CAD build for the part. Positions are in the model's coordinates, mm. Coordinates: 2 decimals unless noted, no trailing zeros. Loops run counter-clockwise (first coordinate to the right, second up) from the corner with the lowest first, then second, coordinate; pieces in that order, holes last. Notation, with made-up numbers: (44, 4) -> (86, 4) arc R7 cw to (86, 13) -> close; hole circle Ø6 at (46, 85.25). An arc over 180 degrees is marked (long way). Write item = value, one per line. Start each with the question number.
(1) Drill centre lines: line 1 (X direction, y = 2.3, z = 0); line 2 (Z direction, x = -1, y = 2.5); line 3 (Z direction, x = -0.25, y = 3.65). Where is each one in solid material? Low to high. Write a range as from..to.
(2) Band-saw the part on B-B (z = 0). Write the cut outline in (x, y).
(3) Band-saw the part on C-C (y = 0.55). Write the cut outline in (x, z).
(4) Band-saw the part on D-D (y = 1.75). Write the cut outline in (x, z), and give its area (3 significant figures).
(5) Flat gauge pins, fed straight in: P1, Ø1.5, axis at x = 1.5, y = 2.5, coming from the +Z side; P2, Ø1, axis at x = -2, y = 2.5, coming from the -Z side. Where does each tip first touch, or does it go through?
(6) Band-saw the part on A-A (x = 0). Write the cut outline in (y, z).
(7) Pull direction X, two halves, no side cores. Call faces 1 (the face through (0.45, 2.92, -1.43)), 2 (the face through (-1.4, 2.98, -3.37)): +X half, -X half, draft (parallel to the pull), parting line (faces both ways), or undercut.
```python
from build123d import *


with BuildPart() as part:
    # Sketch1 → Revolve1 (revolve)
    with BuildSketch(Plane.XY, mode=Mode.PRIVATE) as revolve1_sk:
        with BuildLine():
            Line((1.5, 4.9), (1.5, 1))
            ThreePointArc((1.5, 1), (1.792893219, 0.292893219), (2.5, 0))
            Line((2.5, 0), (2.65, 0))
            ThreePointArc((2.65, 0), (3.357106781, 0.292893219), (3.65, 1))
            Line((3.65, 1), (3.65, 4.9))
            ThreePointArc((3.65, 4.9), (3.357106781, 5.607106781), (2.65, 5.9))
            Line((2.65, 5.9), (2.5, 5.9))
            ThreePointArc((2.5, 5.9), (1.792893219, 5.607106781), (1.5, 4.9))
        make_face()
    revolve(revolve1_sk.sketch.rotate(Axis((0, 5.902912508, 0), (0, -1, 0)), 270), axis=Axis((0, 5.902912508, 0), (0, -1, 0)))


solid = part.part
```
Findings below:
q1.line_1 = -3.65..-1.5, 1.5..3.65
q1.line_2 = -3.51..-1.12, 1.12..3.51
q1.line_3 = -3.64..-1.48, 1.48..3.64
q2.outline = (-3.65, 1) arc R1 ccw to (-2.65, 0) -> (-2.5, 0) arc R1 ccw to (-1.5, 1) -> (-1.5, 4.9) arc R1 ccw to (-2.5, 5.9) -> (-2.65, 5.9) arc R1 ccw to (-3.65, 4.9) -> close; (1.5, 1) arc R1 ccw to (2.5, 0) -> (2.65, 0) arc R1 ccw to (3.65, 1) -> (3.65, 4.9) arc R1 ccw to (2.65, 5.9) -> (2.5, 5.9) arc R1 ccw to (1.5, 4.9) -> close
q3.outline = circle Ø7.09 at (0, 0); hole circle Ø3.21 at (0, 0)
q4.outline = circle Ø7.3 at (0, 0); hole circle Ø3 at (0, 0)
q4.area = 34.8 mm²
q5.P1 = 3.57
q5.P2 = -3.33
q6.outline = (0, -2.65) arc R1 ccw to (1, -3.65) -> (4.9, -3.65) arc R1 ccw to (5.9, -2.65) -> (5.9, -2.5) arc R1 ccw to (4.9, -1.5) -> (1, -1.5) arc R1 ccw to (0, -2.5) -> close; (0, 2.5) arc R1 ccw to (1, 1.5) -> (4.9, 1.5) arc R1 ccw to (5.9, 2.5) -> (5.9, 2.65) arc R1 ccw to (4.9, 3.65) -> (1, 3.65) arc R1 ccw to (0, 2.65) -> close
q7.face_1 = undercut
q7.face_2 = parting line
